from build123d import *

# Parameters (mm, degrees)
F1_DEPTH = 3.81
F2_T     = -1.27
F3_R     = 1.27


with BuildPart() as f1:
    # F0 (on Top) → F1 (new body)
    with BuildSketch(Plane.XY):
        with BuildLine():
            ThreePointArc((22.86, 6.35), (22.116051, 8.146051), (20.32, 8.89))
            Line((20.32, 8.89), (-20.32, 8.89))
            ThreePointArc((-20.32, 8.89), (-22.116051, 8.146051), (-22.86, 6.35))
            Line((-22.86, 6.35), (-22.86, -6.35))
            ThreePointArc((-22.86, -6.35), (-22.116051, -8.146051), (-20.32, -8.89))
            Line((-20.32, -8.89), (20.32, -8.89))
            ThreePointArc((20.32, -8.89), (22.116051, -8.146051), (22.86, -6.35))
            Line((22.86, -6.35), (22.86, 6.35))
        make_face()
    extrude(amount=F1_DEPTH)

    # F2
    f2_openings = [f1.faces().sort_by_distance(p)[0] for p in [
        (0, 0, 3.81),
    ]]
    offset(amount=F2_T, openings=f2_openings)

    # F3
    f3_edges = [f1.edges().sort_by_distance(p)[0] for p in [
        (0, -8.89, 0),
    ]]
    fillet(f3_edges, radius=F3_R)


solid = f1.part
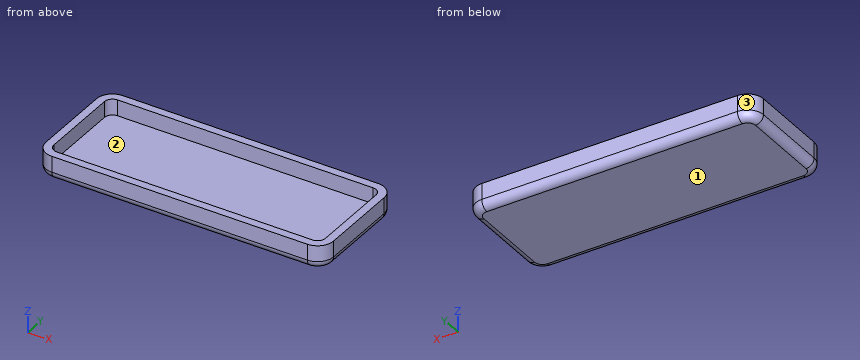
The listing builds one solid part. Answer for the finished solid, in the listing's coordinates (mm). Face numbers are marked on the shaded views. Give positions to 0.01 mm unless a question says otherwise; leave off trailing zeros. Write each loop counter-clockwise with the first axis right and the second up, starting at its lowest first coordinate (ties: lowest second). Pieces come first, ordered by that corner, then holes. Notation, with made-up numbers: (12.25, 22) - (51.25, 22) arc R19 cw to (51.25, 47) - close; hole circle Ø11 at (39, 17.5). An arc over 180 degrees is marked (long way). Use a Markdown table: item, result.
1. Each of these flat-tipped pins is pushed along its axis until it touches: P1, Ø1, axis at x = 1, y = -3, coming from the +Z side; P2, Ø7.5, axis at x = -5.5, y = -4, coming from the +Z side. Where does it stop, or does it pass through?
Values follow:
| item | result |
|---|---|
| P1 | stops at z = 1.27 |
| P2 | stops at z = 3.81 |
2. Find the intervals of material crossed by probe 1 along Y at (x, z) = (17, 2.3); probe 2 along X at (y, z) = (1, 2.25); probe 3 along Z at (x, y) = (9.5, 3.5), in increasing order. Write a range as from..to.
Values follow:
| item | result |
|---|---|
| probe 1 | y = -8.89..-7.62, 7.62..8.89 |
| probe 2 | x = -22.86..-21.59, 21.59..22.86 |
| probe 3 | z = 0..1.27 |
3. For a pull along Y with two mould halves and no side action, classify the marked faces 1, 2 and 3 as released by +Y, released by -Y, zero draft, split by the parting line, or undercut.
Values follow:
| item | result |
|---|---|
| face 1 | zero draft |
| face 2 | undercut |
| face 3 | released by +Y |
4. Section A-A on z = 2.4 is taken. Write down the section's boundary in (x, y), plus the area to 3 significant figures.
Values follow:
| item | result |
|---|---|
| outline | (-22.86, -6.35) arc R2.54 ccw to (-20.32, -8.89) - (20.32, -8.89) arc R2.54 ccw to (22.86, -6.35) - (22.86, 6.35) arc R2.54 ccw to (20.32, 8.89) - (-20.32, 8.89) arc R2.54 ccw to (-22.86, 6.35) - close; hole (-21.59, -6.35) arc R1.27 ccw to (-20.32, -7.62) - (20.32, -7.62) arc R1.27 ccw to (21.59, -6.35) - (21.59, 6.35) arc R1.27 ccw to (20.32, 7.62) - (-20.32, 7.62) arc R1.27 ccw to (-21.59, 6.35) - close |
| area | 151 mm² |
5. Section C-C on x = -13 is taken. Write down the section's boundary in (y, z), plus the area to 3 significant figures.
Values follow:
| item | result |
|---|---|
| outline | (-8.89, 1.27) arc R1.27 ccw to (-7.62, 0) - (7.62, 0) arc R1.27 ccw to (8.89, 1.27) - (8.89, 3.81) - (7.62, 3.81) - (7.62, 1.27) - (-7.62, 1.27) - (-7.62, 3.81) - (-8.89, 3.81) - close |
| area | 28.3 mm² |
6. Section B-B on y = 5.75 is taken. Write down the section's boundary in (x, z), plus the area to 3 significant figures.
Values follow:
| item | result |
|---|---|
| outline | (-22.86, 1.27) arc R1.27 ccw to (-21.59, 0) - (21.59, 0) arc R1.27 ccw to (22.86, 1.27) - (22.86, 3.81) - (21.59, 3.81) - (21.59, 1.27) - (-21.59, 1.27) - (-21.59, 3.81) - (-22.86, 3.81) - close |
| area | 63.8 mm² |
